Could you check a few things on this drawing? It's one solid part, dimensions in mm from its lowest x, y, z. Give positions to 0.01 mm unless a question says otherwise; leave off trailing zeros. Order: outer loops, then holes, each group sorted by start corner. A loop starts at its lowest first (then second) coordinate and runs counter-clockwise, first axis right, second up. Notation, with made-up numbers: (-33.5, 57.25) -> (21.5, 57.25) arc R36 ccw to (21.5, 91.25) -> close; hole circle Ø7 at (25, -20). An arc over 180 degrees is marked (long way). Answer as a JSON object with one key per item and string values.
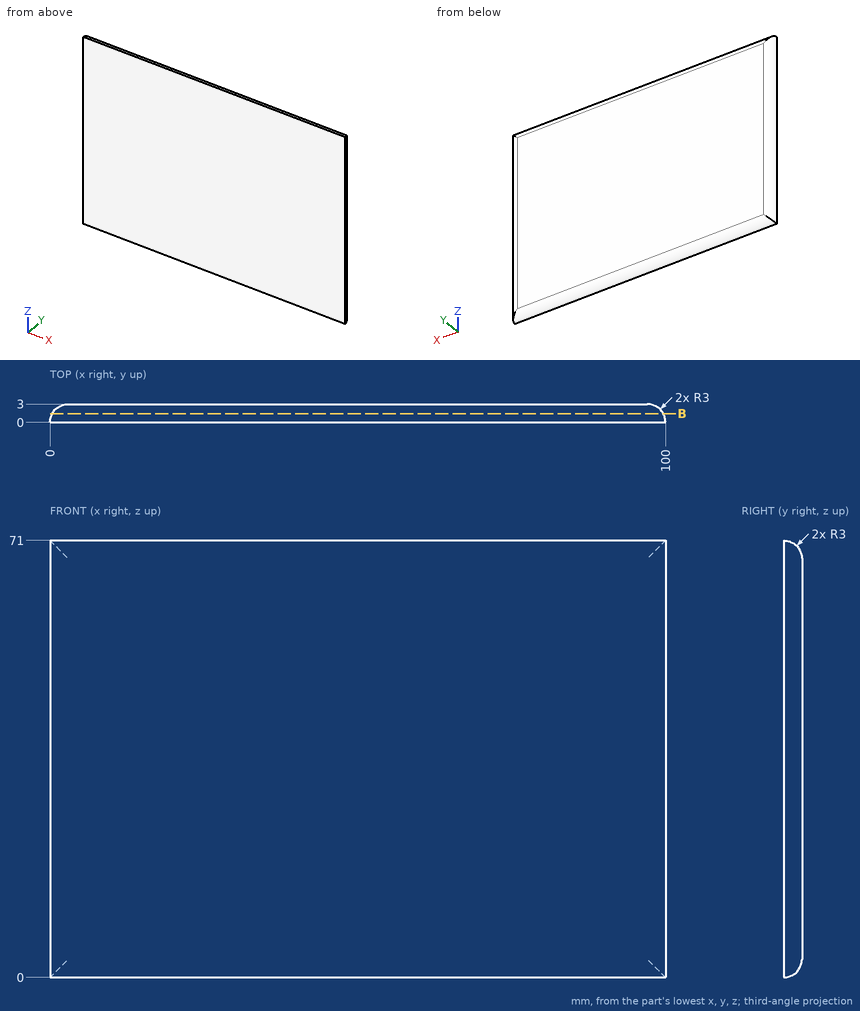
1. If we section it at B-B on y = 1.45: Please give me the cut outline in (x, z).
Worked answers:
{"outline": "(0.37, 0.37) -> (99.63, 0.37) -> (99.63, 70.63) -> (0.37, 70.63) -> close"}
2. Will this pin go through, and if not, where does the flat tip stop? pin 1 Ø1.5 at (y, z) = (1, 59) entering from -X.
Worked answers:
{"pin 1": "x = 0.01"}
3. Please list where these lines run through material, in increasing order: L1, parallel to Z at x = 21.5, y = 0.15; L2, parallel to Z at x = 60.5, y = 2.7; L3, parallel to X at y = 0.65, z = 32.
Worked answers:
{"L1": "0 to 71", "L2": "1.69 to 69.31", "L3": "0.07 to 99.93"}
